from build123d import *

# Parameters (mm, degrees)
F0_R          = 6
F0_R_2        = 0.9
F1_DEPTH      = 5
F3_R          = 6
F3_R_2        = 0.9
F4_DEPTH      = 5
F5_W          = 5
F5_H          = 80
F6_DEPTH      = 63
F6_DEPTH_BACK = 17
F7_R          = 5
F8_R          = 3


with BuildPart() as f1:
    # F0 (on Top) → F1 (new body)
    with BuildSketch(Plane.XY):
        Circle(F0_R)
        Circle(F0_R_2, mode=Mode.SUBTRACT)
    extrude(amount=F1_DEPTH)



with BuildPart() as f4:
    # F3 (on offset) → F4 (new body)
    with BuildSketch(Plane.XY.offset(46)):
        Circle(F3_R)
        Circle(F3_R_2, mode=Mode.SUBTRACT)
    extrude(amount=-F4_DEPTH)


with BuildPart() as f1_1:
    add(f1.part)

    add(f4.part)  # F6 merges F4
    # F5 (on Top) → F6 (join, two sides)
    with BuildSketch(Plane.XY) as f6_sk:
        with Locations((8.4999, 40.012752)):
            Rectangle(F5_W, F5_H)
    extrude(amount=F6_DEPTH)
    extrude(f6_sk.sketch, amount=-F6_DEPTH_BACK)

    # F7
    f7_edges = [f1_1.edges().sort_by_distance(p)[0] for p in [
        (5.9999, 0.034641, 43.5),
        (5.9999, 0.034641, 2.5),
        (5.999986, 0.012752, 2.5),
        (5.999986, 0.012752, 43.5),
    ]]
    fillet(f7_edges, radius=F7_R)

    # F8
    f8_edges = [f1_1.edges().sort_by_distance(p)[0] for p in [
        (8.4999, 80.012752, 63),
        (8.4999, 0.012752, 63),
        (8.4999, 80.012752, -17),
        (8.4999, 0.012752, -17),
    ]]
    fillet(f8_edges, radius=F8_R)


solid = f1_1.part
Geometry check sheet. Reference: the model listing, model coordinates, mm. Round coordinates to 2 decimals unless told otherwise and drop trailing zeros. Order: outer loops, then holes, each group sorted by start corner. A loop starts at its lowest first (then second) coordinate and runs counter-clockwise, first axis right, second up. Notation, with made-up numbers: M -9.75,81 L 34.25,81 A16 ccw 34.25,106 Z; hole C 85.5,77 d6. An arc over 180 degrees is marked long. Answer in a Markdown table with one row per item. Add a question column.
Item 1: Sectioned sample at C-C, the plane z = 25. Enter the section's corners in (x, y).
Item 2: Sectioned sample at D-D, the plane y = 7. Enter the section's corners in (x, z), plus the area to 3 significant figures.
Item 3: Sectioned sample at B-B, the plane y = 34. Enter the section's corners in (x, z), plus the area to 3 significant figures.
Item 4: Draft check along Z on faces 1 (the face through (2, 1, 41)), 2 (the face through (4.41, 7.3, 2.46)), 3 (the face through (8.535, 79.111, 62.145)), 4 (the face through (8.53, 0.91, -16.14)). Enter one of: released by +Z, released by -Z, zero draft, split by the parting line, or undercut.
Item 5: Depth check by flat-ended pin: pin 1 Ø2 at (x, y) = (0, 0) entering from -Z; pin 2 Ø2.5 at (x, y) = (0, 0) entering from +Z; pin 3 Ø4.5 at (x, y) = (6, 0.5) entering from +Z; pin 4 Ø8 at (x, y) = (5, -0.5) entering from -Z. Enter the tip coordinate at first touch or a pass-through.
Item 6: Sectioned sample at A-A, the plane x = 7.5. Enter the section's corners in (y, z).
Item 7: Material ranges on L1, parallel to Y at x = 0, z = 2.4; L2, parallel to X at y = 60, z = 20; L3, parallel to Y at x = 8.5, z = 50, recorded low to high. Write a range as [from, to].
Filled in:
| question | item | result |
|---|---|---|
| 1 | outline | M 6,0.01 L 11,0.01 L 11,80.01 L 6,80.01 Z |
| 2 | outline | M 4.06,0 L 6,0 L 6,-17 L 11,-17 L 11,63 L 6,63 L 6,46 L 4.06,46 L 4.06,41 L 6,41 L 6,5 L 4.06,5 Z |
| 2 | area | 419 mm² |
| 3 | outline | M 6,-17 L 11,-17 L 11,63 L 6,63 Z |
| 3 | area | 400 mm² |
| 4 | face 1 | undercut |
| 4 | face 2 | zero draft |
| 4 | face 3 | released by +Z |
| 4 | face 4 | released by -Z |
| 5 | pin 1 | stops at z = 0 |
| 5 | pin 2 | stops at z = 46 |
| 5 | pin 3 | stops at z = 62.99 |
| 5 | pin 4 | stops at z = -17 |
| 6 | outline | M -0.55,0 L 0.01,0 L 0.01,-14 A3 ccw 3.01,-17 L 77.01,-17 A3 ccw 80.01,-14 L 80.01,60 A3 ccw 77.01,63 L 3.01,63 A3 ccw 0.01,60 L 0.01,46 L -0.55,46 L -0.55,41 L 0.01,41 L 0.01,5 L -0.55,5 Z |
| 7 | L1 | y = [-6, -0.9], [0.9, 6] |
| 7 | L2 | x = [6, 11] |
| 7 | L3 | y = [0.01, 80.01] |
